Job drawing, mm, ordinate dimensions from the low corner. One solid piece. A direction names the side the tool comes from. Round coordinates to 2 decimals unless told otherwise and drop trailing zeros. Write each loop counter-clockwise with the first axis right and the second up, starting at its lowest first coordinate (ties: lowest second). Pieces come first, ordered by that corner, then holes.
1) Saw through at B-B (x = 5). Write the cut outline in (y, z).
2) Saw through at A-A (z = 12.5). Write the cut outline in (x, y), plus the area to 3 significant figures.
3) Wall check: probe 1 along Z at (x, y) = (0.35, 5); probe 2 along Y at (x, z) = (6, 10.5). Give the ranges that are in metal, low to high.
4) Saw through at D-D (z = 6.75). Write the cut outline in (x, y), plus the area to 3 significant figures.
5) Which spindle directions (+Z, -Z, +X, -X, +Y, -Y) get a long thin tool onto all of the face, cutting with end or side? Do the marked faces 1 and 2. Say none if no direction does.
6) Flat gauge pins, fed straight in: pin 1 (2.5 mm diameter, centred on x = 6.5, z = 10, fed in from +Y); pin 2 (2.5 mm diameter, centred on y = 5, z = 2.5, fed in from +X). Where does each tip first touch, or does it go through?
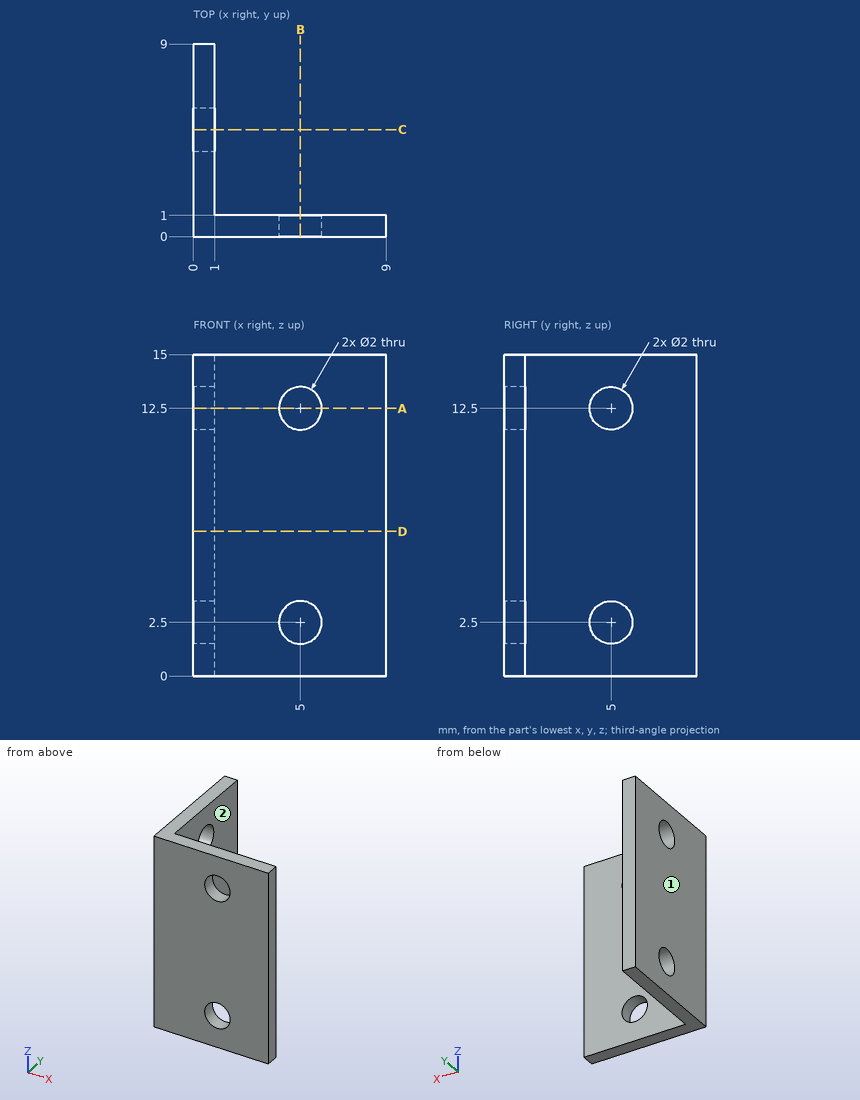
Evaluation:
1. outline: (0, 0) - (1, 0) - (1, 1.5) - (0, 1.5) - close; (0, 3.5) - (1, 3.5) - (1, 11.5) - (0, 11.5) - close; (0, 13.5) - (1, 13.5) - (1, 15) - (0, 15) - close
2. outline: (0, 0) - (4, 0) - (4, 1) - (1, 1) - (1, 4) - (0, 4) - close; (0, 6) - (1, 6) - (1, 9) - (0, 9) - close; (6, 0) - (9, 0) - (9, 1) - (6, 1) - close
2. area: 13.0 mm2
3. probe 1: z = 0 to 1.5, 3.5 to 11.5, 13.5 to 15
3. probe 2: y = 0 to 1
4. outline: (0, 0) - (9, 0) - (9, 1) - (1, 1) - (1, 9) - (0, 9) - close
4. area: 17.0 mm2
5. face 1: +Z, -Z, -X, +Y, -Y
5. face 2: +Z, -Z, +X, +Y
6. pin 1: stops at y = 1
6. pin 2: stops at x = 1
